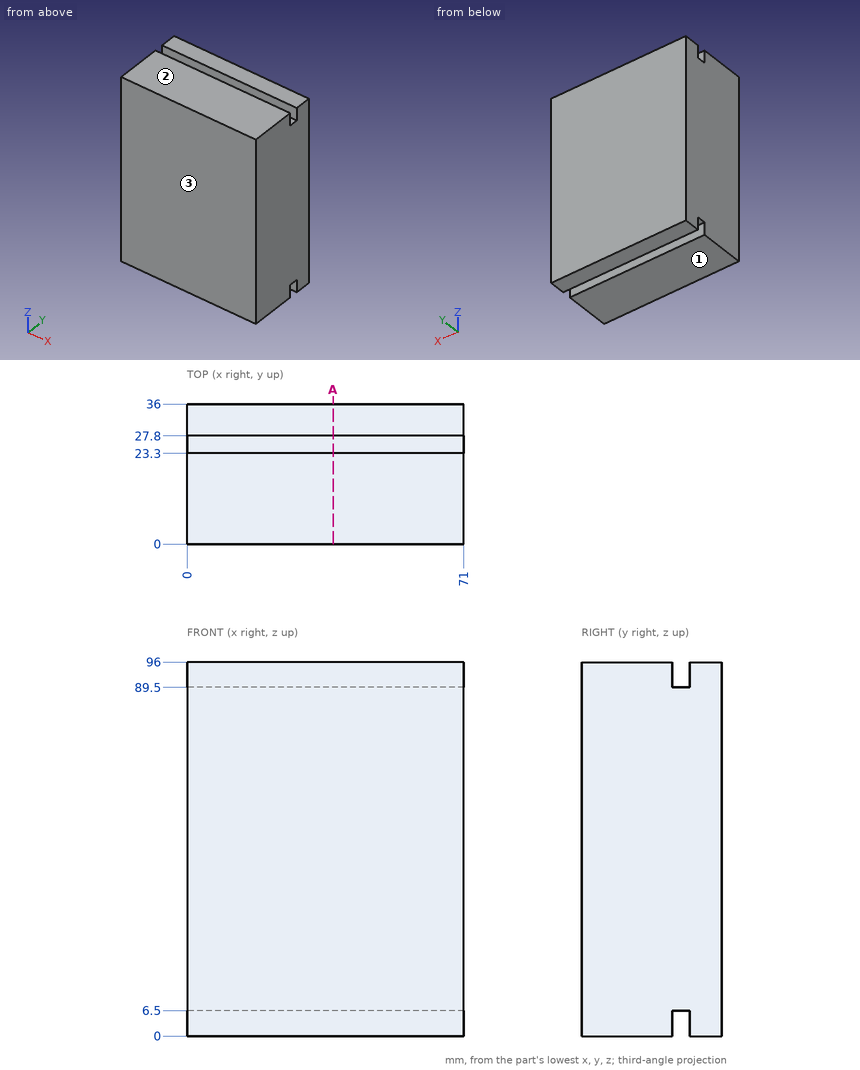
Print and shaded views of the part. All mm, measured from the part's lowest x, y and z. Give positions to 0.01 mm unless a question says otherwise; leave off trailing zeros. Write each loop counter-clockwise with the first axis right and the second up, starting at its lowest first coordinate (ties: lowest second). Pieces come first, ordered by that corner, then holes. Notation, with made-up numbers: M -20,88.25 L -13,88.25 A26 cw -13,106.25 Z; hole C 15,87 d11. An arc over 180 degrees is marked long. Use a Markdown table: item, result.
1) Pull direction Z, two halves, no side cores. Call the marked faces 1, 2 and 3: +Z half, -Z half, draft (parallel to the pull), parting line (faces both ways), or undercut.
Responses:
| item | result |
|---|---|
| face 1 | -Z half |
| face 2 | +Z half |
| face 3 | draft |
2) Cut at A-A (x = 37.5). List the corners of the cut face in (y, z), and give its area (3 significant figures).
Responses:
| item | result |
|---|---|
| outline | M 0,0 L 23.3,0 L 23.3,6.5 L 27.8,6.5 L 27.8,0 L 36,0 L 36,96 L 27.8,96 L 27.8,89.5 L 23.3,89.5 L 23.3,96 L 0,96 Z |
| area | 3,400 mm2 |
3) Pin check, flat tips, straight feed: pin 1 (3.5 mm diameter, centred on x = 43.5, y = 25, fed in from -Z); pin 2 (2 mm diameter, centred on x = 29.5, y = 26.5, fed in from +Z). Stop position of each tip, or through.
Responses:
| item | result |
|---|---|
| pin 1 | stops at z = 0 |
| pin 2 | stops at z = 89.5 |
4) Drill centre line: line 1 (Z direction, x = 41.5, y = 27). Where is it in solid material? Low to high. Write a range as from..to.
Responses:
| item | result |
|---|---|
| line 1 | z = 6.5..89.5 |
